Here's the drawing with two shaded views (mm, measured from the low corner). I have some questions. Round coordinates to 2 decimals unless told otherwise and drop trailing zeros. Loops run counter-clockwise (first coordinate to the right, second up) from the corner with the lowest first, then second, coordinate; pieces in that order, holes last.
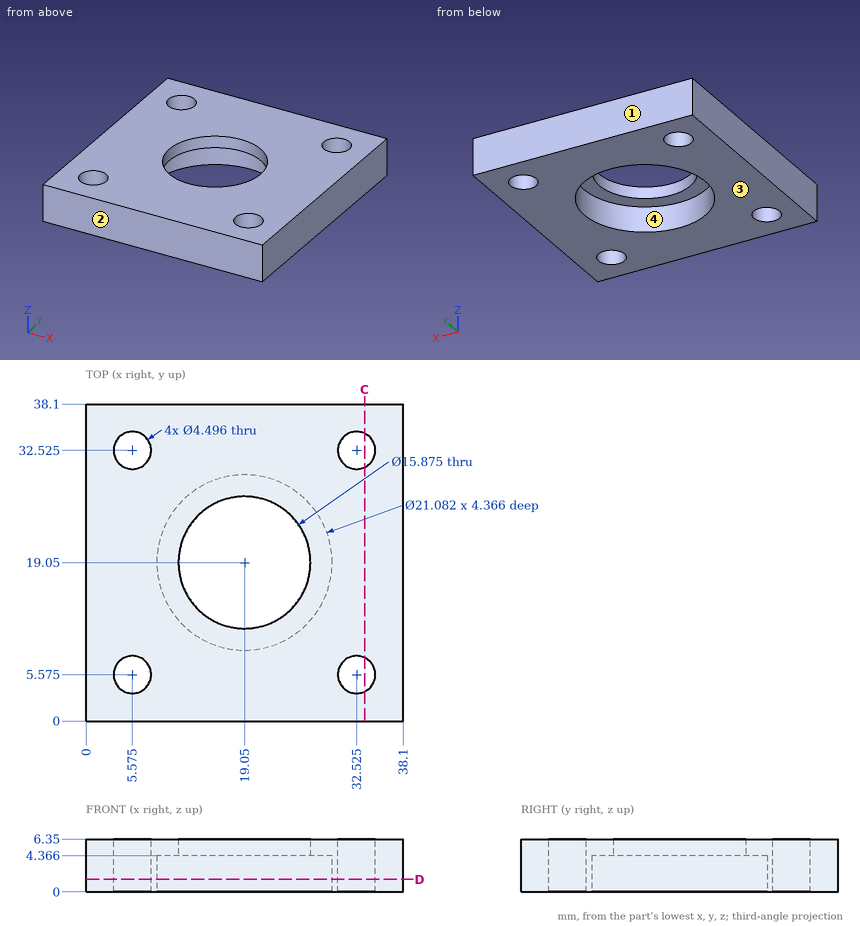
Item 1: We'd pull the mould along Y, two halves only. Please class the marked faces 1, 2, 3 and 4: released by +Y, released by -Y, zero draft, split by the parting line, or undercut.
Results list:
face 1: released by +Y
face 2: released by -Y
face 3: zero draft
face 4: undercut
Item 2: If I drill on line 1 along Y through (x, z) = (5.5, 4.25); line 2 along Y through (x, z) = (19.05, 5.35); line 3 along Y through (x, z) = (6.5, 5.5) (1 decimal), over which ranges is the centre line in solid material (lowest first)?
Results list:
line 1: y = 0 to 3.33, 7.82 to 30.28, 34.77 to 38.1
line 2: y = 0 to 11.11, 26.99 to 38.1
line 3: y = 0 to 3.5, 7.6 to 30.5, 34.6 to 38.1
Item 3: If we section it at D-D, the plane z = 1.5: Count the separate pieces of the cut face and the enclosed holes in it, then the cut area to 3 significant figures.
Results list:
separate pieces: 1
enclosed holes: 5
area: 1,040 mm2
Item 4: If we section it at C-C, the plane x = 33.5: Please give me the cut outline in (y, z).
Results list:
outline: (0, 0) - (3.55, 0) - (3.55, 6.35) - (0, 6.35) - close; (7.6, 0) - (30.5, 0) - (30.5, 6.35) - (7.6, 6.35) - close; (34.55, 0) - (38.1, 0) - (38.1, 6.35) - (34.55, 6.35) - close
